Can you work these out from the drawing? Everything is in mm from the part's minimum corner. A direction names the side the tool comes from. Round coordinates to 2 decimals unless told otherwise and drop trailing zeros. Write each loop counter-clockwise with the first axis right and the second up, starting at its lowest first coordinate (ties: lowest second). Pieces come first, ordered by that corner, then holes. Notation, with made-up numbers: (84.5, 86) -> (115.5, 86) arc R31 ccw to (115.5, 123) -> close; hole circle Ø10 at (20, 79.25). An arc over 180 degrees is marked (long way). Answer as CSV lines item,"result". Start each with the question number.
Q1. Will these pins go through, and if not, where does the flat tip stop? pin 1 Ø2 at (x, y) = (19, 4) entering from -Z; pin 2 Ø1.6 at (y, z) = (17.5, 1) entering from -X; pin 3 Ø1.6 at (y, z) = (12.5, 0.5) entering from +X.
Q2. Imagine slicing it at B-B on y = 21.25. Please give me the cut outline in (x, z), and give its area (3 significant figures).
Q3. If we mould it in two halves opening along X, with no side actions, what happens to the marked faces 1, 2, 3 and 4? For each: pulls with the +X half, pulls with the -X half, needs draft (parallel to the pull), parting line crosses it, or undercut.
Q4. Imagine slicing it at C-C on z = 18. Please give me the cut outline in (x, y).
Q5. Imagine slicing it at D-D on x = 24. Please give me the cut outline in (y, z), and give its area (3 significant figures).
Q6. For the marked faces 5, 6 and 7, which set-ups out of +Z, -Z, +X, -X, +Y, -Y let a thin tool reach every point of the face, with its end or its side?
Q7. If I drill on line 1 (X direction, y = 25.5, z = 26); line 2 (Z direction, x = 23.1, y = 15); line 3 (Z direction, x = 21.25, y = 15.5), over which ranges is the centre line in solid material (lowest first)? Write a range as [from, to].
Q8. Imagine slicing it at A-A on x = 12.7. Please give me the cut outline in (y, z).
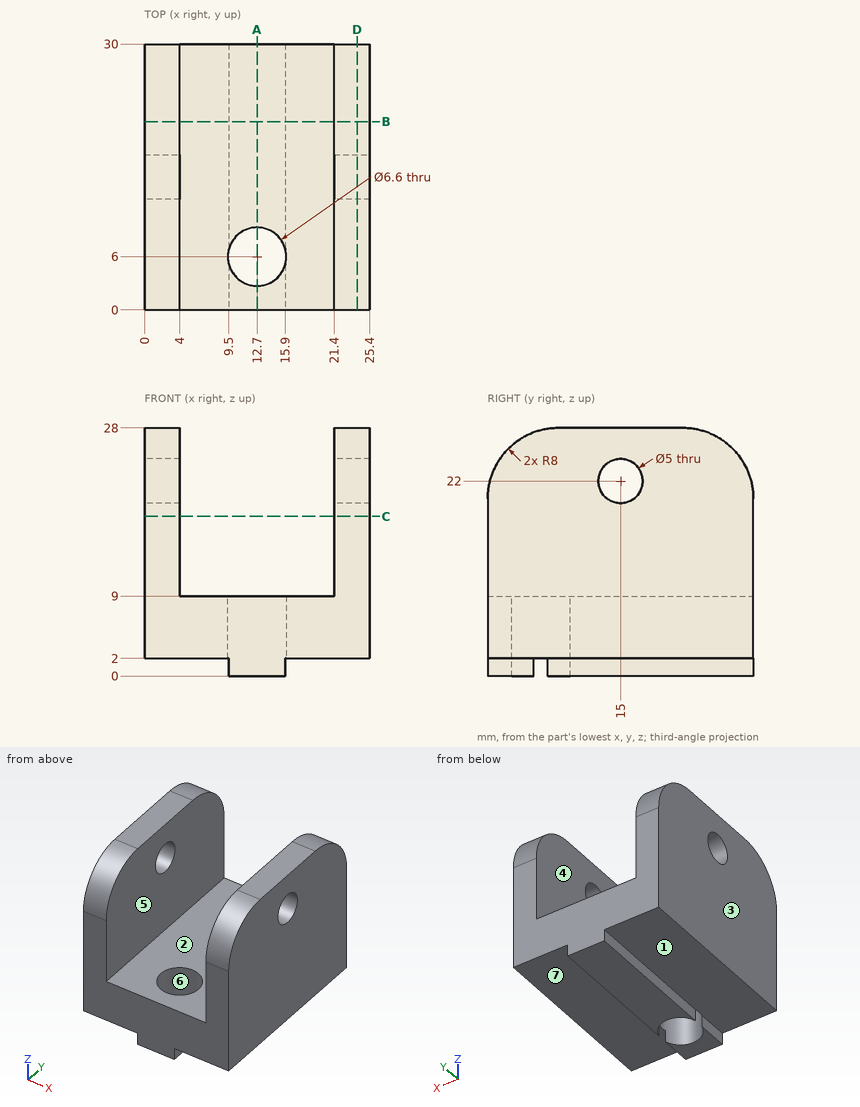
Checks:
1,pin 1,"z = 2"
1,pin 2,"x = 9.5"
1,pin 3,"x = 15.9"
2,outline,"(0, 2) -> (9.5, 2) -> (9.5, 0) -> (15.9, 0) -> (15.9, 2) -> (25.4, 2) -> (25.4, 28) -> (21.4, 28) -> (21.4, 9) -> (4, 9) -> (4, 28) -> (0, 28) -> close"
2,area,"343 mm^2"
3,face 1,"needs draft"
3,face 2,"undercut"
3,face 3,"pulls with the -X half"
3,face 4,"undercut"
4,outline,"(0, 0) -> (4, 0) -> (4, 30) -> (0, 30) -> close; (21.4, 0) -> (25.4, 0) -> (25.4, 30) -> (21.4, 30) -> close"
5,outline,"(0, 2) -> (30, 2) -> (30, 20) arc R8 ccw to (22, 28) -> (8, 28) arc R8 ccw to (0, 20) -> close; hole circle Ø5 at (15, 22)"
5,area,"733 mm^2"
6,face 5,"+Z, +Y, -Y"
6,face 6,"+Z, -Z"
6,face 7,"-Z, +X, +Y, -Y"
7,line 1,"[0, 4], [21.4, 25.4]"
7,line 2,"[2, 19.5], [24.5, 28]"
7,line 3,"[2, 9]"
8,outline,"(0, 0) -> (2.7, 0) -> (2.7, 9) -> (0, 9) -> close; (9.3, 0) -> (30, 0) -> (30, 9) -> (9.3, 9) -> close"
